Design review of the part built by this model. Coordinates are the model's own, in mm. A direction names the side the tool comes from. Give positions to 0.01 mm unless a question says otherwise; leave off trailing zeros. Write each loop counter-clockwise with the first axis right and the second up, starting at its lowest first coordinate (ties: lowest second). Pieces come first, ordered by that corner, then holes.
Autodesk Inventor part; units mm, degrees
ref_plane "YZ Plane" through (0, 0, 0) normal (1, 0, 0) x (0, 1, 0)
ref_plane "XZ Plane" through (0, 0, 0) normal (0, 1, 0) x (-1, 0, 0)
ref_plane "XY Plane" through (0, 0, 0) normal (0, 0, 1) x (1, 0, 0)
sketch "Sketch1" plane through (0, 0, 0) normal (0, 1, 0) x (-1, 0, 0)
  line L0 (0, 0) -> (10.5, 0) construction
  line L1 (0, 0) -> (0, -171.8) construction
  line L2 (0, -171.8) -> (47.15, -171.8) construction
  line L3 (0, -21.8) -> (9.5, -21.8) construction
  line L4 (0, -20.8) -> (9.5, -20.8) construction
  line L5 (0, -15.3) -> (12.6, -15.3) construction
  line L6 (8, 0) -> (10.5, 0)
  line L7 (10.5, 0) -> (10.5, -15.3)
  line L8 (10.5, -15.3) -> (12.6, -15.3)
  line L9 (12.6, -15.3) -> (9.5, -20.8)
  line L10 (9.5, -20.8) -> (9.5, -21.8)
  line L11 (8, 0) -> (8, -21.8)
  arc A0 (9.5, -21.8) -> (47.15, -171.8) centre (327.1298, -21.8) ccw
  arc A1 (8, -21.8) -> (45.4494, -171.8) centre (327.1298, -21.8) ccw
  arc A2 (45.4494, -171.8) -> (47.15, -171.8) centre (46.2997, -171.3472) ccw
  dimension "d0" = 150
  dimension "d1" = 1
  dimension "d2" = 5.5
  dimension "d3" = 15.3
  dimension "d4" = 47.15
  dimension "d5" = 9.5
  dimension "d6" = 9.5
  dimension "d7" = 12.6
  dimension "d8" = 10.5
  dimension "d9" = 1.5
revolve "Revolution1" add sketch "Sketch1" angle 360 about axis through (0, 0, 0) along (0, 0, -1)
thread "Thread1"
equation "\"d0\" = Flare_Length"
equation "\"d1\" = Transition_Length"
equation "\"d2\" = Mount_Flange_Length"
equation "\"d3\" = Mount_Length"
equation "\"d4\" = Flare_Diameter"
equation "\"d6\" = Tail_Diameter"
equation "\"d7\" = Mount_Flange_Diameter"
equation "\"d8\" = Mount_Diameter"
equation "\"d9\" = Bell_Thickness"
equation "\"Transition_Length\" = 1"
properties part number "Horn_D" material "Steel, Cast"
(1) Consider section A-A, the plane y = 0. Give the boundary of the cut face in (x, z), then the cut area to 3 significant figures.
Resolved:
outline: (-47.15, -171.8) arc R0.96 ccw to (-45.45, -171.8) arc R319.13 ccw to (-8, -21.8) - (-8, 0) - (-10.5, 0) - (-10.5, -15.3) - (-12.6, -15.3) - (-9.5, -20.8) - (-9.5, -21.8) arc R317.63 cw to start; (8, -21.8) arc R319.13 ccw to (45.45, -171.8) arc R0.96 ccw to (47.15, -171.8) arc R317.63 cw to (9.5, -21.8) - (9.5, -20.8) - (12.6, -15.3) - (10.5, -15.3) - (10.5, 0) - (8, 0) - close
area: 583 mm2
(2) Consider section D-D, the plane z = -51. Give the boundary of the cut face in (x, y).
Resolved:
outline: circle Ø21.69 at (0, 0); hole circle Ø18.68 at (0, 0)
(3) To check wall thickness, follow L1, parallel to Y at x = 0, z = -15; L2, parallel to Y at x = 0, z = -17; L3, parallel to X at y = -0.5, z = -17. State the ranges of each line that lie inside material, in increasing order.
Resolved:
L1: y = -10.5 to -8, 8 to 10.5
L2: y = -11.64 to -8, 8 to 11.64
L3: x = -11.63 to -7.98, 7.98 to 11.63
(4) Mouldability with a two-part tool opening along Y and no side actions: class faces 3 (the face through (1.26, -9.61, -20.46)), 4 (the face through (1.73, -7.81, -11.05)), 5 (the face through (2, -8, 0)) as pulls with the +Y half, pulls with the -Y half, needs draft (parallel to the pull), parting line crosses it, or undercut.
Resolved:
face 3: parting line crosses it
face 4: undercut
face 5: needs draft
(5) Clearance check with flat-ended pins moving along their axes: P1, Ø6, axis at x = 21.5, z = -117, coming from the +Y side; P2, Ø2, axis at x = 1, y = 13.5, coming from the +Z side; P3, Ø1.5, axis at x = -30, y = -4, coming from the -Z side. State where each tip first meets the part, or that it passes through.
Resolved:
P1: stops at y = 15.74
P2: stops at z = -15.3
P3: stops at z = -140.8
(6) Consider section C-C, the plane z = -13. Give the boundary of the cut face in (x, y), then the cut area to 3 significant figures.
Resolved:
outline: circle Ø21 at (0, 0); hole circle Ø16 at (0, 0)
area: 145 mm2
(7) Tool access review of faces 1 (the face through (2.9, 10.3, -15.3)), 2 (the face through (-4.38, -8.43, -21.31)): name each direction out of +Z, -Z, +X, -X, +Y, -Y from which nothing blocks a thin tool from reaching the whole face with its end or side.
Resolved:
face 1: +Z
face 2: none
